Read the model definition and answer for the solid it produces. Units are mm, in the model's axes. A direction names the side the tool comes from. Give positions to 0.01 mm unless a question says otherwise; leave off trailing zeros. Write each loop counter-clockwise with the first axis right and the second up, starting at its lowest first coordinate (ties: lowest second). Pieces come first, ordered by that corner, then holes. Notation, with made-up numbers: (13, 78.5) -> (56, 78.5) arc R22 cw to (56, 92.5) -> close; hole circle Ø4 at (6, 31.5). An arc over 180 degrees is marked (long way). Answer as CSV lines item,"result". Start each with the question number.
1. Find the intervals of material crossed by line 1 (X direction, y = -9.5, z = -35); line 2 (X direction, y = -16.5, z = -27.5); line 3 (Y direction, x = 30, z = -44), in increasing order.
2. The part is cut by section D-D, the plane x = 28. Determine the outline of the cut face in (y, z), and give its area (3 significant figures).
3. The part is cut by section C-C, the plane z = -53.5. Determine the outline of the cut face in (x, y).
4. The part is cut by section B-B, the plane y = -42. Determine the outline of the cut face in (x, z), and give its area (3 significant figures).
5. Given pin 1 (3.5 mm diameter, centred on x = 61.5, y = -33.5, fed in from +Z); pin 2 (8 mm diameter, centred on y = -29.5, z = -57, fed in from +X); pin 3 (0.5 mm diameter, centred on x = 67.5, y = -8, fed in from -Z), each flat-ended and moving along its own axis, determine where each tip first touches the part or whether it passes through.
6. The part is cut by section A-A, the plane z = -4. Determine the outline of the cut face in (x, y), and give its area (3 significant figures).
7. A tool of negligible diameter and unlimited length cuts with its end or side. For faces 5 (the flat face through (61, -31, -50.701)), 6 (the flat face through (17.142, -6, -26)), from which of +Z, -Z, +X, -X, +Y, -Y can it reach the whole face along a straight path? Write none if from no direction.
8. For a pull along X with two mould halves and no side action, classify faces 1 (the flat face through (16.878, -31, -26)), 2 (the flat face through (0, -31, -31)), 3 (the flat face through (67.942, -6, -26)), 4 (the flat face through (9, -31, 0)) as pulls with the +X half, pulls with the -X half, needs draft (parallel to the pull), parting line crosses it, or undercut.
from build123d import *

# Parameters (mm, degrees)
F0_W     = 38.1
F0_H     = 12.7
F1_DEPTH = 63.5
F2_W     = 10.787756
F2_H     = 12.239977
F3_DEPTH = 25.4
F5_W     = 12.7
F5_H     = 12.7
F6_DEPTH = 50.8
F7_W     = 50.8
F7_H     = 50.8
F8_DEPTH = 12.7


with BuildPart() as f1:
    # F0 (on Front) → F1 (new body)
    with BuildSketch(Plane.XZ):
        Polygon((16.877607, 0), (0, 0), (0, -63.5), (16.877607, -63.5), (16.877607, -63.351139), (16.877607, -50.651139), align=None)
        with Locations((35.927607, -57.001139)):
            Rectangle(F0_W, F0_H)
    extrude(amount=F1_DEPTH)

    # F5 (on Front) → F6 (join)
    with BuildSketch(Plane.XZ):
        with Locations((60.988158, -57.050698)):
            Rectangle(F5_W, F5_H)
    extrude(amount=F6_DEPTH)

    # F7 (on Front) → F8 (join)
    with BuildSketch(Plane.XZ):
        with Locations((42.542354, -25.4)):
            Rectangle(F7_W, F7_H)
    extrude(amount=F8_DEPTH)


with BuildPart() as f3:
    # F2 (on Front) → F3 (new body)
    with BuildSketch(Plane.XZ):
        with Locations((60.992375, -56.739516)):
            Rectangle(F2_W, F2_H)
    extrude(amount=F3_DEPTH)


solid = f1.part
Results found:
1,line 1,"x = 0 to 16.88, 17.14 to 67.94"
1,line 2,"x = 0 to 16.88"
1,line 3,"y = -12.7 to 0"
2,outline,"(-63.5, -63.35) -> (0, -63.35) -> (0, 0) -> (-12.7, 0) -> (-12.7, -50.65) -> (-63.5, -50.65) -> close"
2,area,"1,450 mm²"
3,outline,"(0, -63.5) -> (54.98, -63.5) -> (54.98, -50.8) -> (67.34, -50.8) -> (67.34, 0) -> (0, 0) -> close"
4,outline,"(0, -63.5) -> (16.88, -63.5) -> (16.88, -63.35) -> (54.64, -63.35) -> (54.64, -63.4) -> (67.34, -63.4) -> (67.34, -50.7) -> (54.98, -50.7) -> (54.98, -50.65) -> (16.88, -50.65) -> (16.88, 0) -> (0, 0) -> close"
4,area,"1,710 mm²"
5,pin 1,"stops at z = -50.7"
5,pin 2,"stops at x = 67.34"
5,pin 3,"stops at z = -63.4"
6,outline,"(0, -63.5) -> (16.88, -63.5) -> (16.88, 0) -> (0, 0) -> close; (17.14, -12.7) -> (67.94, -12.7) -> (67.94, 0) -> (17.14, 0) -> close"
6,area,"1,720 mm²"
7,face 5,"+Z, +X, -Y"
7,face 6,"+Z, +Y, -Y"
8,face 1,"undercut"
8,face 2,"pulls with the -X half"
8,face 3,"pulls with the +X half"
8,face 4,"needs draft"
